Build history of the part. All positions in model axes, mm. Round coordinates to 2 decimals unless told otherwise and drop trailing zeros. Write each loop counter-clockwise with the first axis right and the second up, starting at its lowest first coordinate (ties: lowest second). Pieces come first, ordered by that corner, then holes.
Item 1: Band-saw the part on A-A, the plane y = 0. Write the cut outline in (x, z).
Item 2: Wall check: probe 1 along Y at (x, z) = (0, 0.7); probe 2 along Y at (x, z) = (-20.5, 1.3); probe 3 along Y at (x, z) = (-11.5, 2.05). Give the ranges that are in metal, low to high.
Item 3: Band-saw the part on D-D, the plane x = -15. Write the cut outline in (y, z), then the cut area to 3 significant figures.
Item 4: Band-saw the part on C-C, the plane z = 1.1. Count the separate pieces of the cut face and the enclosed holes in it, then the cut area to 3 significant figures.
Item 5: Drop a flat-ended pin along its axis: pin 1 Ø4 at (x, y) = (21.21, -21.21) entering from -Z. Give the stop position or say it passes through.
```python
from build123d import *

# Parameters (mm, degrees)
F0_R     = 2.55
F0_R_2   = 1.6
F0_R_3   = 7.5
F1_DEPTH = 3.14


with BuildPart() as f1:
    # F0 (on Top) → F1 (new body)
    with BuildSketch(Plane.XY):
        with BuildLine():
            ThreePointArc((-17.854446, 24.571961), (-24.571961, 24.571961), (-24.571961, 17.854446))
            Line((-24.571961, 17.854446), (-20.793457, 14.075942))
            ThreePointArc((-20.793457, 14.075942), (-19.813844, 12.163673), (-20.136055, 10.039386))
            ThreePointArc((-20.136055, 10.039386), (-22.5, 0), (-20.136055, -10.039386))
            ThreePointArc((-20.136055, -10.039386), (-19.813844, -12.163673), (-20.793457, -14.075942))
            Line((-20.793457, -14.075942), (-24.571961, -17.854446))
            ThreePointArc((-24.571961, -17.854446), (-24.571961, -24.571961), (-17.854446, -24.571961))
            Line((-17.854446, -24.571961), (-14.075942, -20.793457))
            ThreePointArc((-14.075942, -20.793457), (-12.163673, -19.813844), (-10.039386, -20.136055))
            ThreePointArc((-10.039386, -20.136055), (0, -22.5), (10.039386, -20.136055))
            ThreePointArc((10.039386, -20.136055), (12.163673, -19.813844), (14.075942, -20.793457))
            Line((14.075942, -20.793457), (17.854446, -24.571961))
            ThreePointArc((17.854446, -24.571961), (24.571961, -24.571961), (24.571961, -17.854446))
            Line((24.571961, -17.854446), (20.793457, -14.075942))
            ThreePointArc((20.793457, -14.075942), (19.813844, -12.163673), (20.136055, -10.039386))
            ThreePointArc((20.136055, -10.039386), (22.5, 0), (20.136055, 10.039386))
            ThreePointArc((20.136055, 10.039386), (19.813844, 12.163673), (20.793457, 14.075942))
            Line((20.793457, 14.075942), (24.571961, 17.854446))
            ThreePointArc((24.571961, 17.854446), (24.571961, 24.571961), (17.854446, 24.571961))
            Line((17.854446, 24.571961), (14.075942, 20.793457))
            ThreePointArc((14.075942, 20.793457), (12.163673, 19.813844), (10.039386, 20.136055))
            ThreePointArc((10.039386, 20.136055), (0, 22.5), (-10.039386, 20.136055))
            ThreePointArc((-10.039386, 20.136055), (-12.163673, 19.813844), (-14.075942, 20.793457))
            Line((-14.075942, 20.793457), (-17.854446, 24.571961))
        make_face()
        with Locations((-21.213203, -21.213203)):
            Circle(F0_R, mode=Mode.SUBTRACT)
        with Locations((-10.606602, -10.606602)):
            Circle(F0_R_2, mode=Mode.SUBTRACT)
        with Locations((21.213203, -21.213203)):
            Circle(F0_R, mode=Mode.SUBTRACT)
        with Locations((10.606602, -10.606602)):
            Circle(F0_R_2, mode=Mode.SUBTRACT)
        Circle(F0_R_3, mode=Mode.SUBTRACT)
        with Locations((-10.606602, 10.606602)):
            Circle(F0_R_2, mode=Mode.SUBTRACT)
        with Locations((-21.213203, 21.213203)):
            Circle(F0_R, mode=Mode.SUBTRACT)
        with Locations((10.606602, 10.606602)):
            Circle(F0_R_2, mode=Mode.SUBTRACT)
        with Locations((21.213203, 21.213203)):
            Circle(F0_R, mode=Mode.SUBTRACT)
    extrude(amount=F1_DEPTH)


solid = f1.part
```
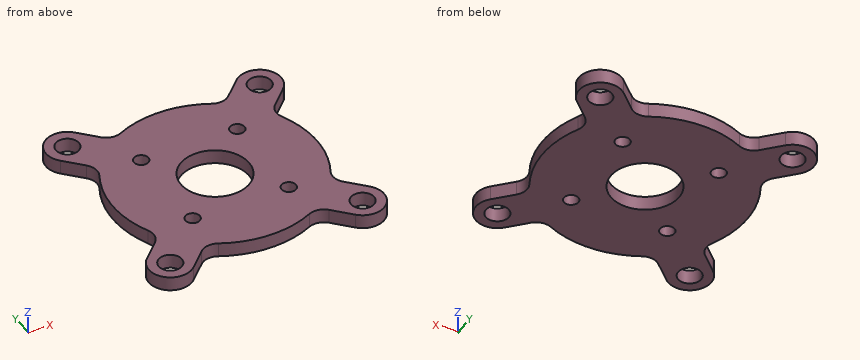
Results:
1. outline: (-22.5, 0) - (-7.5, 0) - (-7.5, 3.14) - (-22.5, 3.14) - close; (7.5, 0) - (22.5, 0) - (22.5, 3.14) - (7.5, 3.14) - close
2. probe 1: y = -22.5 to -7.5, 7.5 to 22.5
2. probe 2: y = -25.91 to -23.66, -18.76 to -13.74, -9.27 to 9.27, 13.74 to 18.76, 23.66 to 25.91
2. probe 3: y = -19.77 to -11.93, -9.28 to 9.28, 11.93 to 19.77
3. outline: (-21.72, 0) - (21.72, 0) - (21.72, 3.14) - (-21.72, 3.14) - close
3. area: 136 mm2
4. separate pieces: 1
4. enclosed holes: 9
4. area: 1,740 mm2
5. pin 1: passes through
